Read the model definition and answer for the solid it produces. Units are mm, in the model's axes. A direction names the side the tool comes from. Coordinates: 2 decimals unless noted, no trailing zeros. Order: outer loops, then holes, each group sorted by start corner. A loop starts at its lowest first (then second) coordinate and runs counter-clockwise, first axis right, second up. Notation, with made-up numbers: M 56,-10.5 L 106,-10.5 A10 cw 106,-1.5 Z; hole C -5.75,86 d10. An arc over 180 degrees is marked long. Use a Markdown table: item, result. Add a question column.
1) Find the intervals of material crossed by probe 1 along Z at (x, y) = (207.5, 759); probe 2 along Y at (x, z) = (194, -165.5); probe 3 along X at (y, z) = (761, 13.5), in increasing order. Write a range as [from, to].
2) Each of these flat-tipped pins is pushed along its axis until it touches: pin 1 Ø12 at (x, z) = (202, 96) entering from +Y; pin 2 Ø10 at (y, z) = (763.5, 3.5) entering from -X; pin 3 Ø3 at (x, y) = (211.88, 716.29) entering from +Z; pin 4 Ø1 at (x, z) = (219, 73.5) entering from -Y. Where does it stop, or does it pass through?
3) Find section A-A on z = -184.5. Write down the section's boundary in (x, y), plus the area to 3 significant figures.
4) For faces 4 (the face through (225.91, 723.436, 226.185)), 5 (the face through (229, 743, 223.838)), 6 (the face through (229, 743, -228.6)), determine the directions among +Z, -Z, +X, -X, +Y, -Y from which every point of the face is accessible in a straight line to the end or side of a thin tool.
5) The mould has two halves that part along Y. Classify faces 1 (the face through (219, 725, -223.838)), 2 (the face through (211.069, 753.135, -226.252)), 3 (the face through (183.79, 750.44, -1.07)): released by +Y, released by -Y, zero draft, split by the parting line, or undercut.
from build123d import *

# Parameters (mm, degrees)
BASE_FLANGE1_DEPTH = 50.8
FILLET1_R          = 4.7625
SKETCH18_R         = 2.4892
CUT_EXTRUDE1_DEPTH = 620.376518124
SKETCH20_R         = 2.4892
CUT_EXTRUDE2_DEPTH = 935.779827906
LPATTERN1_START    = -228.6
LPATTERN1_DEPTH    = 457.2


# Read off the part's stored shape, not the designer's step: LPattern1
# Sheet-metal steps are written as plain solids
with BuildPart() as part:
    # Sketch17 → Base-Flange1 (new body)
    with BuildSketch(Plane(origin=(494.7314495, 252.078264185, 0), x_dir=(0, 0, -1), z_dir=(0.8910065241883655, 0.4539904997395516, 0))):
        with BuildLine():
            Line((-228.6, 533.849573814), (-228.6, 582.300073814))
            ThreePointArc((-228.6, 582.300073814), (-226.981911413, 586.206485227), (-223.0755, 587.824573814))
            Line((-223.0755, 587.824573814), (223.0755, 587.824573814))
            ThreePointArc((223.0755, 587.824573814), (226.981911413, 586.206485227), (228.6, 582.300073814))
            Line((228.6, 582.300073814), (228.6, 533.849573814))
            Line((228.6, 533.849573814), (223.8375, 533.849573814))
            Line((223.8375, 533.849573814), (223.8375, 582.300073814))
            ThreePointArc((223.8375, 582.300073814), (223.614315367, 582.838889181), (223.0755, 583.062073814))
            Line((223.0755, 583.062073814), (-223.0755, 583.062073814))
            ThreePointArc((-223.0755, 583.062073814), (-223.614315367, 582.838889181), (-223.8375, 582.300073814))
            Line((-223.8375, 582.300073814), (-223.8375, 533.849573814))
            Line((-223.8375, 533.849573814), (-228.6, 533.849573814))
        make_face()
    extrude(amount=-BASE_FLANGE1_DEPTH)

    # Fillet1
    fillet1_edges = [part.edges().sort_by_distance(p)[0] for p in [
        (252.368814698, 727.741717389, -226.21875),
        (252.368814698, 727.741717389, 226.21875),
        (207.105683269, 704.679000002, -226.21875),
        (207.105683269, 704.679000002, 226.21875),
    ]]
    fillet(fillet1_edges, radius=FILLET1_R)

    # Sketch18 → Cut-Extrude1 (cut, through all)
    with BuildSketch(Plane(origin=(-264.70464227, 519.512111775, 0), x_dir=(0.8910065241883653, 0.4539904997395517, 0), z_dir=(0.4539904997395517, -0.8910065241883653, 0))):
        with Locations((536.200086356, -196.85)):
            Circle(SKETCH18_R)
        with Locations((548.900086356, -196.85)):
            Circle(SKETCH18_R)
        with Locations((523.500086356, -196.85)):
            Circle(SKETCH18_R)
        with Locations((510.800086356, -196.85)):
            Circle(SKETCH18_R)
    cut_extrude1 = extrude(amount=-CUT_EXTRUDE1_DEPTH, mode=Mode.SUBTRACT)

    # Mirror1: Cut-Extrude1 across plane
    add(cut_extrude1.mirror(Plane.XY), mode=Mode.SUBTRACT)

    # Sketch20 → Cut-Extrude2 (cut, through all)
    with BuildSketch(Plane(origin=(0, 0, -228.6), x_dir=(-1, 0, 0), z_dir=(0, 0, -1))):
        with Locations((-240.170605262, 730.70143613)):
            Circle(SKETCH20_R)
        with Locations((-232.963506079, 744.846164702)):
            Circle(SKETCH20_R)
        with Locations((-204.674048936, 730.431966335)):
            Circle(SKETCH20_R)
        with Locations((-211.881148119, 716.287237764)):
            Circle(SKETCH20_R)
        with Locations((-197.466949753, 744.576694907)):
            Circle(SKETCH20_R)
        with Locations((-225.756406896, 758.990893273)):
            Circle(SKETCH20_R)
        with BuildLine():
            Line((-235.084869956, 726.089937384), (-218.601249184, 717.691113101))
            ThreePointArc((-218.601249184, 717.691113101), (-217.902023556, 715.539117896), (-220.054018761, 714.839892268))
            Line((-220.054018761, 714.839892268), (-236.537639533, 723.238716552))
            ThreePointArc((-236.537639533, 723.238716552), (-237.236865161, 725.390711756), (-235.084869956, 726.089937384))
        make_face()
    extrude(amount=-CUT_EXTRUDE2_DEPTH, mode=Mode.SUBTRACT)

    # LPattern1 outline → LPattern1 (cut)
    with BuildSketch(Plane.XY.offset(LPATTERN1_START)):
        with BuildLine():
            ThreePointArc((200.441629536, 753.331373399), (199.742403908, 751.179378195), (201.894399112, 750.480152566))
            Line((201.894399112, 750.480152566), (218.378019885, 758.878976849))
            ThreePointArc((218.378019885, 758.878976849), (219.077245513, 761.030972054), (216.925250308, 761.730197682))
            Line((216.925250308, 761.730197682), (200.441629536, 753.331373399))
        make_face()
        with BuildLine():
            ThreePointArc((202.711581992, 748.876340861), (202.012356364, 746.724345657), (204.164351568, 746.025120028))
            Line((204.164351568, 746.025120028), (220.647972341, 754.423944312))
            ThreePointArc((220.647972341, 754.423944312), (221.347197969, 756.575939517), (219.195202764, 757.275165145))
            Line((219.195202764, 757.275165145), (202.711581992, 748.876340861))
        make_face()
        with BuildLine():
            ThreePointArc((204.981534448, 744.421308324), (204.28230882, 742.26931312), (206.434304024, 741.570087491))
            Line((206.434304024, 741.570087491), (222.917924797, 749.968911775))
            ThreePointArc((222.917924797, 749.968911775), (223.617150425, 752.12090698), (221.46515522, 752.820132607))
            Line((221.46515522, 752.820132607), (204.981534448, 744.421308324))
        make_face()
        with BuildLine():
            ThreePointArc((207.251486904, 739.966275787), (206.552261276, 737.814280582), (208.704256481, 737.115054954))
            Line((208.704256481, 737.115054954), (225.187877253, 745.513879237))
            ThreePointArc((225.187877253, 745.513879237), (225.887102881, 747.665874442), (223.735107676, 748.36510007))
            Line((223.735107676, 748.36510007), (207.251486904, 739.966275787))
        make_face()
        with BuildLine():
            ThreePointArc((209.52143936, 735.51124325), (208.822213732, 733.359248045), (210.974208937, 732.660022417))
            Line((210.974208937, 732.660022417), (227.457829709, 741.0588467))
            ThreePointArc((227.457829709, 741.0588467), (228.157055337, 743.210841905), (226.005060132, 743.910067533))
            Line((226.005060132, 743.910067533), (209.52143936, 735.51124325))
        make_face()
        with BuildLine():
            ThreePointArc((211.791391816, 731.056210713), (211.092166188, 728.904215508), (213.244161393, 728.20498988))
            Line((213.244161393, 728.20498988), (229.727782165, 736.603814163))
            ThreePointArc((229.727782165, 736.603814163), (230.427007793, 738.755809368), (228.275012588, 739.455034996))
            Line((228.275012588, 739.455034996), (211.791391816, 731.056210713))
        make_face()
        with BuildLine():
            ThreePointArc((214.061344272, 726.601178175), (213.362118644, 724.44918297), (215.514113849, 723.749957343))
            Line((215.514113849, 723.749957343), (231.997734621, 732.148781626))
            ThreePointArc((231.997734621, 732.148781626), (232.696960249, 734.300776831), (230.544965044, 735.000002459))
            Line((230.544965044, 735.000002459), (214.061344272, 726.601178175))
        make_face()
        with BuildLine():
            ThreePointArc((216.331296728, 722.146145638), (215.6320711, 719.994150433), (217.784066305, 719.294924805))
            Line((217.784066305, 719.294924805), (234.267687077, 727.693749089))
            ThreePointArc((234.267687077, 727.693749089), (234.966912705, 729.845744294), (232.8149175, 730.544969922))
            Line((232.8149175, 730.544969922), (216.331296728, 722.146145638))
        make_face()
    extrude(amount=LPATTERN1_DEPTH, mode=Mode.SUBTRACT)


solid = part.part
Check result:
| question | item | result |
|---|---|---|
| 1 | probe 1 | z = [-228.6, -223.84], [223.84, 228.6] |
| 1 | probe 2 | y = [753.23, 758.58] |
| 1 | probe 3 | x = [198.75, 209.24] |
| 2 | pin 1 | stops at y = 765.71 |
| 2 | pin 2 | stops at x = 193.85 |
| 2 | pin 3 | passes through |
| 2 | pin 4 | stops at y = 765.72 |
| 3 | outline | M 182.6,752.77 L 184.76,748.53 L 230.03,771.59 L 227.86,775.83 Z |
| 3 | area | 242 mm2 |
| 4 | face 4 | +Z, -Z |
| 4 | face 5 | +X, -Y |
| 4 | face 6 | -Z, +X, -X, +Y, -Y |
| 5 | face 1 | zero draft |
| 5 | face 2 | undercut |
| 5 | face 3 | released by -Y |
